Work out the finished part from the listing and answer in its coordinate system (mm). Face numbers are marked on the shaded views. A direction names the side the tool comes from. Give positions to 0.01 mm unless a question says otherwise; leave off trailing zeros. Order: outer loops, then holes, each group sorted by start corner. A loop starts at its lowest first (then second) coordinate and runs counter-clockwise, first axis right, second up.
```python
from build123d import *

# Parameters (mm, degrees)
SKETCH1_W           = 54
SKETCH1_H           = 28.5
SKETCH1_W_2         = 5
SKETCH1_H_2         = 22.5
SKETCH1_R           = 1.7
SKETCH1_R_2         = 7.5
BOSS_EXTRUDE2_DEPTH = 3
SKETCH2_W           = 4
SKETCH2_H           = 20.5
BOSS_EXTRUDE3_DEPTH = 21.75
SKETCH4_R           = 10.25
BOSS_EXTRUDE4_DEPTH = 4
SKETCH6_R           = 4.4
SKETCH6_R_2         = 1.45
CUT_EXTRUDE3_DEPTH  = 4
SKETCH7_R           = 1.45
CUT_EXTRUDE4_DEPTH  = 1.5
SKETCH8_W           = 28.781481152
SKETCH8_H           = 28.5
BOSS_EXTRUDE5_DEPTH = 3
SKETCH9_R           = 1.7
CUT_EXTRUDE5_DEPTH  = 3


with BuildPart() as part:
    # Sketch1 → Boss-Extrude2 (new body)
    with BuildSketch(Plane(origin=(0, 0, 0), x_dir=(1, 0, 0), z_dir=(0, 1, 0))):
        Rectangle(SKETCH1_W, SKETCH1_H)
        with Locations((20.5, 0)):
            Rectangle(SKETCH1_W_2, SKETCH1_H_2, mode=Mode.SUBTRACT)
        with Locations((-20.5, 0)):
            Rectangle(SKETCH1_W_2, SKETCH1_H_2, mode=Mode.SUBTRACT)
        with Locations(Location((-9, -8.25, 0), (0, 0, 270))):
            Circle(SKETCH1_R, mode=Mode.SUBTRACT)
        with Locations(Location((9, -8.25, 0), (0, 0, 270))):
            Circle(SKETCH1_R, mode=Mode.SUBTRACT)
        with Locations(Location((-9, 8.25, 0), (0, 0, 270))):
            Circle(SKETCH1_R, mode=Mode.SUBTRACT)
        with Locations(Location((0, 0, 0), (0, 0, 270))):
            Circle(SKETCH1_R_2, mode=Mode.SUBTRACT)
        with Locations(Location((9, 8.25, 0), (0, 0, 270))):
            Circle(SKETCH1_R, mode=Mode.SUBTRACT)
    extrude(amount=BOSS_EXTRUDE2_DEPTH)

    # Sketch2 → Boss-Extrude3 (add)
    with BuildSketch(Plane(origin=(0, 3, 0), x_dir=(1, 0, 0), z_dir=(0, 1, 0))):
        with Locations((25, 0)):
            Rectangle(SKETCH2_W, SKETCH2_H)
    boss_extrude3 = extrude(amount=BOSS_EXTRUDE3_DEPTH)

    # Sketch4 → Boss-Extrude4 (add)
    with BuildSketch(Plane(origin=(27, 0, 0), x_dir=(0, 0, -1), z_dir=(1, 0, 0))):
        with Locations((0, 24.75)):
            Circle(SKETCH4_R)
    boss_extrude4 = extrude(amount=-BOSS_EXTRUDE4_DEPTH)

    # Mirror1: Boss-Extrude3, Boss-Extrude4 across plane
    add(boss_extrude3.mirror(Plane(origin=(0, 0, 0), x_dir=(0, 0, 1), z_dir=(1, 0, 0))))
    add(boss_extrude4.mirror(Plane(origin=(0, 0, 0), x_dir=(0, 0, 1), z_dir=(1, 0, 0))))

    # Sketch6 → Cut-Extrude3 (cut)
    with BuildSketch(Plane(origin=(27, 0, 0), x_dir=(0, 0, -1), z_dir=(1, 0, 0))):
        with Locations((0, 24.75)):
            Circle(SKETCH6_R)
        with Locations((0, 32.75)):
            Circle(SKETCH6_R_2)
        with Locations((8, 24.75)):
            Circle(SKETCH6_R_2)
        with Locations((0, 16.75)):
            Circle(SKETCH6_R_2)
        with Locations((-8, 24.75)):
            Circle(SKETCH6_R_2)
    cut_extrude3 = extrude(amount=-CUT_EXTRUDE3_DEPTH, mode=Mode.SUBTRACT)

    # Mirror3: Cut-Extrude3 across plane
    add(cut_extrude3.mirror(Plane(origin=(0, 0, 0), x_dir=(0, 0, 1), z_dir=(1, 0, 0))), mode=Mode.SUBTRACT)

    # Sketch7 → Cut-Extrude4 (cut)
    # profile 1 of 4: a face of its own
    with BuildSketch(Plane(origin=(27, 0, 0), x_dir=(0, 0, -1), z_dir=(1, 0, 0))):
        with BuildLine():
            ThreePointArc((10.25, 24.75), (10.200627247, 25.754840168), (10.052984631, 26.75))
            Line((10.052984631, 26.75), (8, 26.75))
            ThreePointArc((8, 26.75), (6, 24.75), (8, 22.75))
            Line((8, 22.75), (10.25, 22.75))
            Line((10.25, 22.75), (10.25, 24.75))
        make_face()
        with Locations((8, 24.75)):
            Circle(SKETCH7_R, mode=Mode.SUBTRACT)
    # profile 2 of 4: a face of its own
    with BuildSketch(Plane(origin=(27, 0, 0), x_dir=(0, 0, -1), z_dir=(1, 0, 0))):
        with BuildLine():
            Line((2, 32.75), (2, 34.802984631))
            ThreePointArc((2, 34.802984631), (0, 35), (-2, 34.802984631))
            Line((-2, 34.802984631), (-2, 32.75))
            ThreePointArc((-2, 32.75), (0, 30.75), (2, 32.75))
        make_face()
        with Locations((0, 32.75)):
            Circle(SKETCH7_R, mode=Mode.SUBTRACT)
    # profile 3 of 4: a face of its own
    with BuildSketch(Plane(origin=(27, 0, 0), x_dir=(0, 0, -1), z_dir=(1, 0, 0))):
        with BuildLine():
            Line((-8, 26.75), (-10.052984631, 26.75))
            ThreePointArc((-10.052984631, 26.75), (-10.200627247, 25.754840168), (-10.25, 24.75))
            Line((-10.25, 24.75), (-10.25, 22.75))
            Line((-10.25, 22.75), (-8, 22.75))
            ThreePointArc((-8, 22.75), (-6, 24.75), (-8, 26.75))
        make_face()
        with Locations((-8, 24.75)):
            Circle(SKETCH7_R, mode=Mode.SUBTRACT)
    # profile 4 of 4: a face of its own
    with BuildSketch(Plane(origin=(27, 0, 0), x_dir=(0, 0, -1), z_dir=(1, 0, 0))):
        with BuildLine():
            Line((-2, 16.75), (-2, 13.927640071))
            Line((-2, 13.927640071), (2, 13.927640071))
            Line((2, 13.927640071), (2, 16.75))
            ThreePointArc((2, 16.75), (0, 18.75), (-2, 16.75))
        make_face()
        with Locations((0, 16.75)):
            Circle(SKETCH7_R, mode=Mode.SUBTRACT)
    cut_extrude4 = extrude(amount=-CUT_EXTRUDE4_DEPTH, mode=Mode.SUBTRACT)

    # Mirror4: Cut-Extrude4 across plane
    add(cut_extrude4.mirror(Plane(origin=(0, 0, 0), x_dir=(0, 0, 1), z_dir=(1, 0, 0))), mode=Mode.SUBTRACT)

    # Sketch8 → Boss-Extrude5 (add)
    with BuildSketch(Plane(origin=(0, 3, 0), x_dir=(1, 0, 0), z_dir=(0, 1, 0))):
        Rectangle(SKETCH8_W, SKETCH8_H)
    extrude(amount=-BOSS_EXTRUDE5_DEPTH)

    # Sketch9 → Cut-Extrude5 (cut)
    with BuildSketch(Plane(origin=(0, 3, 0), x_dir=(1, 0, 0), z_dir=(0, 1, 0))):
        with BuildLine():
            ThreePointArc((-5.3, -7), (-5.797918472, -5.797918472), (-7, -5.3))
            Line((-7, -5.3), (-7, -7))
            Line((-7, -7), (-5.3, -7))
        make_face()
        with BuildLine():
            Line((-7, -7), (-7, -5.3))
            ThreePointArc((-7, -5.3), (-8.202081528, -8.202081528), (-5.3, -7))
            Line((-5.3, -7), (-7, -7))
        make_face()
        with BuildLine():
            ThreePointArc((8.7, -7), (8.202081528, -5.797918472), (7, -5.3))
            Line((7, -5.3), (7, -7))
            Line((7, -7), (5.3, -7))
            ThreePointArc((5.3, -7), (7, -8.7), (8.7, -7))
        make_face()
        with BuildLine():
            Line((7, -7), (7, -5.3))
            ThreePointArc((7, -5.3), (5.797918472, -5.797918472), (5.3, -7))
            Line((5.3, -7), (7, -7))
        make_face()
        with BuildLine():
            ThreePointArc((8.7, 7), (7, 8.7), (5.3, 7))
            Line((5.3, 7), (7, 7))
            Line((7, 7), (7, 5.3))
            ThreePointArc((7, 5.3), (8.202081528, 5.797918472), (8.7, 7))
        make_face()
        with BuildLine():
            Line((7, 7), (5.3, 7))
            ThreePointArc((5.3, 7), (5.797918472, 5.797918472), (7, 5.3))
            Line((7, 5.3), (7, 7))
        make_face()
        with Locations(Location((-7, 7, 0), (0, 0, 270))):
            Circle(SKETCH9_R)
    extrude(amount=-CUT_EXTRUDE5_DEPTH, mode=Mode.SUBTRACT)


solid = part.part
```
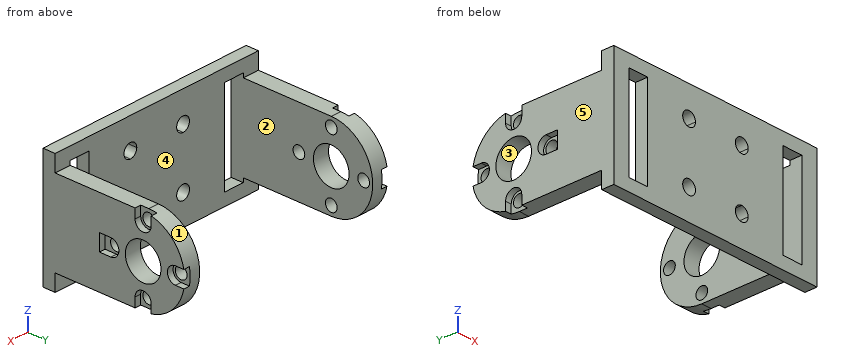
1. The mould has two halves that part along X. Classify the marked faces 3, 4 and 5: pulls with the +X half, pulls with the -X half, needs draft (parallel to the pull), parting line crosses it, or undercut.
Findings below:
face 3: needs draft
face 4: undercut
face 5: pulls with the -X half
2. The part is cut by section C-C (z = 0). State how many separate pieces and enclosed holes the cut face has, then the cut area to 3 significant figures.
Findings below:
separate pieces: 9
enclosed holes: 0
area: 261 mm2
3. The part is cut by section B-B (y = 32). Write down the section's boundary in (x, z).
Findings below:
outline: (-27, -7.25) - (-23, -7.25) - (-23, -1.24) - (-25.5, -1.24) - (-25.5, -1.85) - (-27, -1.85) - close; (-27, 1.85) - (-25.5, 1.85) - (-25.5, 1.24) - (-23, 1.24) - (-23, 7.25) - (-27, 7.25) - close; (23, -7.25) - (27, -7.25) - (27, -1.85) - (25.5, -1.85) - (25.5, -1.24) - (23, -1.24) - close; (23, 1.24) - (25.5, 1.24) - (25.5, 1.85) - (27, 1.85) - (27, 7.25) - (23, 7.25) - close
4. Which of the six approach directions +Z, -Z, +X, -X, +Y, -Y give full straight-line access (tool end or side, diameter ignored) to the marked faces 1 and 2?
Findings below:
face 1: +X, -X, +Y
face 2: +Y, -Y
5. Straight lines are drawn through the part: probe 1 along Y at (x, z) = (24.5, 0); probe 2 along X at (y, z) = (33, 4.5); probe 3 along Y at (x, z) = (12, 2). For each, find the intervals that lie inside material, in ascending order.
Findings below:
probe 1: y = 0 to 15.3, 18.2 to 20.35, 29.15 to 31.3, 34.2 to 35
probe 2: x = -27 to -23, 23 to 27
probe 3: y = 0 to 3
6. The part is cut by section A-A (x = 8). Write down the section's boundary in (y, z), then the cut area to 3 significant figures.
Findings below:
outline: (0, -14.25) - (3, -14.25) - (3, -8.37) - (0, -8.37) - close; (0, -5.63) - (3, -5.63) - (3, 5.63) - (0, 5.63) - close; (0, 8.37) - (3, 8.37) - (3, 14.25) - (0, 14.25) - close
area: 69.0 mm2
7. Given P1, Ø0.8, axis at x = -26.5, y = 33.5, coming from the +Z side; P2, Ø1.6, axis at x = 26, y = 15.5, coming from the -Z side; P3, Ø2.5, axis at y = 24.75, z = -8, coming from the -X side; P4, Ø3.5, axis at y = 24.75, z = -8, coming from the +X side, each flat-ended and moving along its own axis, determine where each tip first touches the part or whether it passes through.
Findings below:
P1: stops at z = 5.94
P2: stops at z = -10.25
P3: passes through
P4: stops at x = 25.5
8. The part is cut by section D-D (x = -17). Write down the section's boundary in (y, z).
Findings below:
outline: (0, -14.25) - (3, -14.25) - (3, 14.25) - (0, 14.25) - close
